Could you check a few things on this drawing? It's one solid part, dimensions in mm from its lowest x, y, z. A direction names the side the tool comes from. Give positions to 0.01 mm unless a question says otherwise; leave off trailing zeros. Order: outer loops, then holes, each group sorted by start corner. A loop starts at its lowest first (then second) coordinate and runs counter-clockwise, first axis right, second up.
(1) Imagine slicing it at C-C, the plane z = 22.25. Write out the boundary of the cut face in (x, y).
(2) If I drill on probe 1 along Y at (x, z) = (48.65, 15); probe 2 along X at (y, z) = (25.5, 12.75); probe 3 along Y at (x, z) = (24, 18), over which ranges is the centre line in solid material (lowest first)?
(3) Will these pins go through, and if not, where does the flat tip stop? pin 1 (1 mm diameter, centred on x = 53, z = 4, fed in from -Y); pin 2 (9 mm diameter, centred on x = 19.5, z = 20, fed in from +Y); pin 3 (4 mm diameter, centred on x = 47.5, y = 5, fed in from -Z); pin 4 (5 mm diameter, centred on x = 18.5, y = 91, fed in from -Z).
(4) Imagine slicing it at B-B, the plane y = 5. Write out the boundary of the cut face in (x, z).
(5) Imagine slicing it at A-A, the plane z = 15. Write out the boundary of the cut face in (x, y), then the cut area to 3 significant figures.
(6) On a 3-axis mill with a long thin cutter (end or side, diameter ignored), from which of +Z, -Z, +X, -X, +Y, -Y can I reach the whole of each face in a straight line? I mean the marked faces 1, 2 and 3. Say none if no direction works.
(7) Imagine slicing it at D-D, the plane x = 14.5. Write out the boundary of the cut face in (y, z), then the cut area to 3 significant figures.
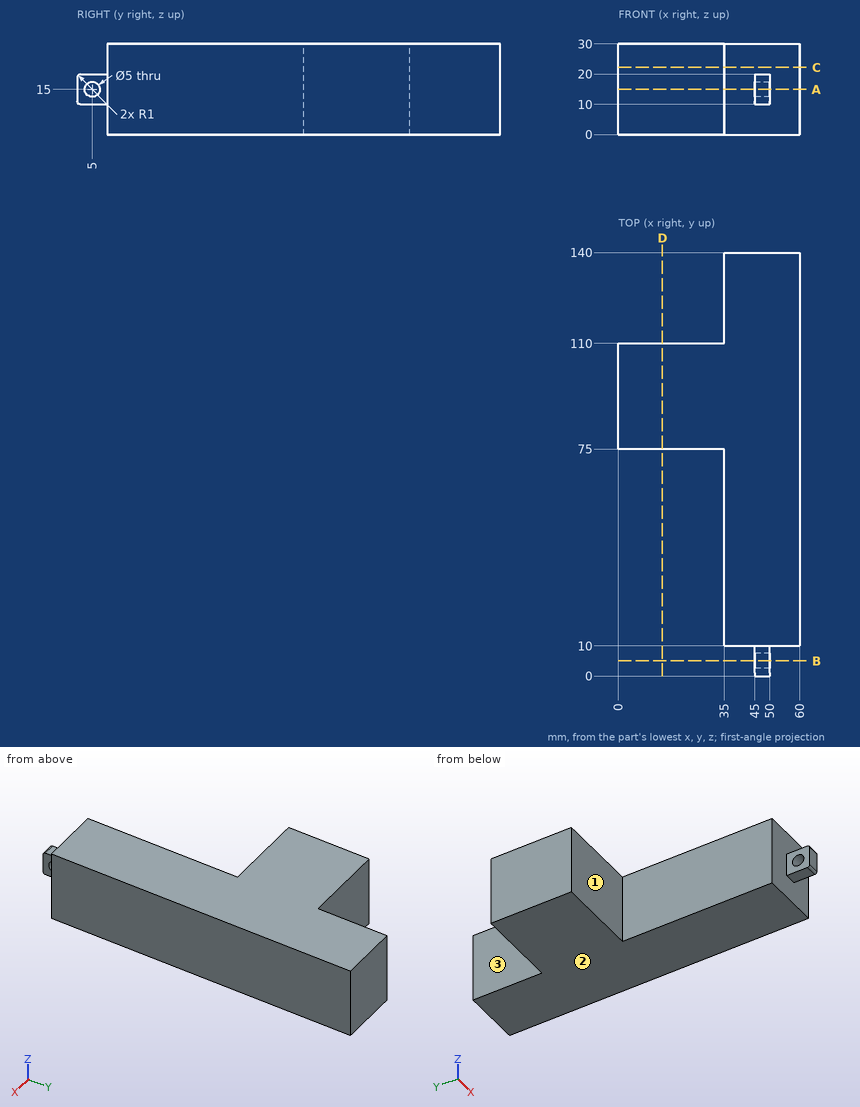
Answer block:
1. outline: (0, 75) - (35, 75) - (35, 10) - (60, 10) - (60, 140) - (35, 140) - (35, 110) - (0, 110) - close
2. probe 1: y = 0 to 2.5, 7.5 to 140
2. probe 2: x = 35 to 60
2. probe 3: y = 75 to 110
3. pin 1: stops at y = 10
3. pin 2: stops at y = 110
3. pin 3: stops at z = 10
3. pin 4: stops at z = 0
4. outline: (45, 10) - (50, 10) - (50, 12.5) - (45, 12.5) - close; (45, 17.5) - (50, 17.5) - (50, 20) - (45, 20) - close
5. outline: (0, 75) - (35, 75) - (35, 10) - (45, 10) - (45, 7.5) - (50, 7.5) - (50, 10) - (60, 10) - (60, 140) - (35, 140) - (35, 110) - (0, 110) - close; (45, 0) - (50, 0) - (50, 2.5) - (45, 2.5) - close
5. area: 4,500 mm2
6. face 1: +Z, -Z, -X, -Y
6. face 2: -Z, +X, -X, +Y, -Y
6. face 3: +Z, -Z, -X, +Y
7. outline: (75, 0) - (110, 0) - (110, 30) - (75, 30) - close
7. area: 1,050 mm2
